Autodesk Inventor part; units mm, degrees
ref_plane "YZ Plane" through (0, 0, 0) normal (1, 0, 0) x (0, 1, 0)
ref_plane "XZ Plane" through (0, 0, 0) normal (0, 1, 0) x (-1, 0, 0)
ref_plane "XY Plane" through (0, 0, 0) normal (0, 0, 1) x (1, 0, 0)
sketch "Sketch1" plane through (0, 0, 0) normal (1, 0, 0) x (0, 1, 0)
  line L0 (0, 0) -> (0, 597.7382)
  line L1 (0, 0) -> (3.175, 0)
  line L2 (3.175, 0) -> (3.175, 594.5632)
  line L3 (3.175, 594.5632) -> (9.906, 594.5632)
  line L4 (9.906, 594.5632) -> (15.756, 595.9828)
  line L5 (0, 597.7382) -> (9.5263, 597.7382)
  line L6 (9.5263, 597.7382) -> (12.7824, 598.5283)
  line L7 (41.2921, 902.0052) -> (15.756, 595.9828)
  line L8 (12.7824, 598.5283) -> (38.1281, 902.2692)
  line L9 (38.1281, 902.2692) -> (41.2921, 902.0052)
  line L10 (41.2921, 902.0052) -> (44.4671, 901.7403)
  line L11 (44.4671, 901.7403) -> (18.7409, 593.44)
  line L12 (18.7409, 593.44) -> (10.2857, 591.3882)
  line L13 (10.2857, 591.3882) -> (6.35, 591.3882)
  line L14 (6.35, 591.3882) -> (6.35, 574.5988)
  line L15 (6.35, 574.5988) -> (3.175, 574.5988)
  line L16 (44.4671, 901.7403) -> (47.6311, 901.4763)
  line L17 (47.6311, 901.4763) -> (21.7146, 590.8944)
  line L18 (21.7146, 590.8944) -> (10.6654, 588.2132)
  line L19 (10.6654, 588.2132) -> (9.525, 588.2132)
  line L20 (9.525, 588.2132) -> (9.525, 432.9684)
  line L21 (9.525, 432.9684) -> (6.35, 432.9684)
  line L22 (6.35, 432.9684) -> (6.35, 574.5988)
  line L23 (32.5862, 759.3601) -> (35.7502, 759.0961)
  point P0 (14.5133, 592.4141)
  dimension "d0" = 594.5632
  dimension "d1" = 3.175
  dimension "d2" = 6.731
  dimension "d7" = 3.175
  dimension "d8" = 6.0198
  dimension "d9" = 166.36
  dimension "d10" = 3.175
  dimension "d11" = 108.41
  dimension "d12" = 3.175
  dimension "d13" = 307.086
  dimension "d18" = 3.175
  dimension "d20" = 307.1025
  dimension "d21" = 8.7006
  dimension "d22" = 3.175
  dimension "d23" = 3.175
  dimension "d24" = 3.9357
  dimension "d25" = 16.7894
  dimension "d28" = 3.175
  dimension "d29" = 3.186
  dimension "d30" = 3.175
  dimension "d32" = 3.175
  dimension "d33" = 3.175
  dimension "d34" = 142.875
  dimension "d35" = 168.7862
  dimension "d36" = 11.3698
  dimension "d37" = 1.1404
  dimension "d38" = 155.2448
extrude "Extrusion3" add sketch "Sketch1" along normal blind 925.83 contours L14 L13 L12 L11 L23 L17 L18 L19 L20 L21 L22
properties part number "Second_Shingle_Over_Intake_Vent_With_Length_36.45_Inches"
The listing builds one solid part. Answer for the finished solid, in the listing's coordinates (mm). A direction names the side the tool comes from. Round coordinates to 2 decimals unless told otherwise and drop trailing zeros. Order: outer loops, then holes, each group sorted by start corner. A loop starts at its lowest first (then second) coordinate and runs counter-clockwise, first axis right, second up. Notation, with made-up numbers: (-26, 12.25) - (-21, 12.25) arc R28 cw to (-21, 39.25) - close; hole circle Ø3 at (-29, 20.25). An arc over 180 degrees is marked (long way). Put each result on its own line as item: value. Start each with the question number.
(1) Given P1, Ø8, axis at x = 456, z = 589.5, coming from the +Y side; P2, Ø4, axis at x = 294, z = 609, coming from the -Y side; P3, Ø12, axis at x = 592.5, z = 716, coming from the +Y side, each flat-ended and moving along its own axis, determine where each tip first touches the part or whether it passes through.
(2) Find section C-C (z = 671). Give the vertices of the cut face in (x, y), plus the area to 3 significant figures.
(3) For faces 1 (the flat face through (456, 9.525, 512)), 2 (the flat face through (0, 20, 597)), determine the directions among +Z, -Z, +X, -X, +Y, -Y from which every point of the face is accessible in a straight line to the end or side of a thin tool.
(4) Find section A-A (z = 457). Give the vertices of the cut face in (x, y) (3 decimals), plus the area to 3 significant figures.
(5) Find section B-B (x = 763.5). Give the vertices of the cut face in (y, z) (3 decimals), plus the area to 3 significant figures.
(6) Straight lines are drawn through the part: probe 1 along Y at (x, z) = (193, 530) (3 decimals); probe 2 along Z at (x, y) = (249.5, 9.25); probe 3 along Z at (x, y) = (253.5, 15.5). For each, find the intervals that lie inside material, in ascending order. Write a range as from..to.
Reply:
1. P1: y = 21.93
1. P2: y = 19.87
1. P3: y = 32.65
2. outline: (0, 25.21) - (925.83, 25.21) - (925.83, 28.4) - (0, 28.4) - close
2. area: 2,950 mm^2
3. face 1: -Z, +X, -X, +Y
3. face 2: +Z, -Z, -X, +Y, -Y
4. outline: (0, 6.35) - (925.83, 6.35) - (925.83, 9.525) - (0, 9.525) - close
4. area: 2,940 mm^2
5. outline: (6.35, 432.968) - (9.525, 432.968) - (9.525, 588.213) - (10.665, 588.213) - (21.715, 590.894) - (35.75, 759.096) - (32.586, 759.36) - (18.741, 593.44) - (10.286, 591.388) - (6.35, 591.388) - close
5. area: 1,070 mm^2
6. probe 1: 6.35..9.525
6. probe 2: 432.97..591.39
6. probe 3: 589.39..592.65
